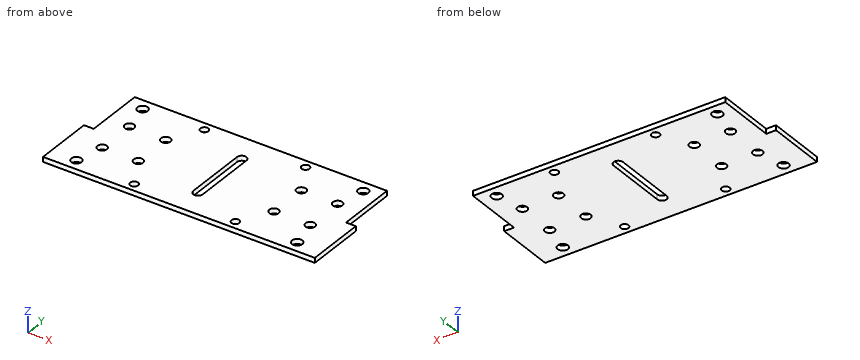
```python
from build123d import *

# Parameters (mm, degrees)
SKETCH1_W           = 160
SKETCH1_H           = 75
BOSS_EXTRUDE1_DEPTH = 3.1
SKETCH2_W           = 6.2
SKETCH2_H           = 37.5
BOSS_EXTRUDE2_DEPTH = 3.1
SKETCH3_R           = 2.5
SKETCH3_R_2         = 3
SKETCH3_R_3         = 3.25
CUT_EXTRUDE1_DEPTH  = 4.1


with BuildPart() as part:
    # Sketch1 → Boss-Extrude1 (new body)
    with BuildSketch(Plane.XY):
        Rectangle(SKETCH1_W, SKETCH1_H)
    extrude(amount=BOSS_EXTRUDE1_DEPTH)

    # Sketch2 → Boss-Extrude2 (add, through all)
    with BuildSketch(Plane.XY.offset(3.1)):
        with Locations((83.1, -18.75)):
            Rectangle(SKETCH2_W, SKETCH2_H)
        with Locations((-83.1, -18.75)):
            Rectangle(SKETCH2_W, SKETCH2_H)
    extrude(amount=-BOSS_EXTRUDE2_DEPTH)

    # Sketch3 → Cut-Extrude1 (cut, through all)
    with BuildSketch(Plane.XY.offset(3.1)):
        with Locations((32.08959236, 32.08959236)):
            Circle(SKETCH3_R)
        with Locations((32.08959236, -32.08959236)):
            Circle(SKETCH3_R)
        with Locations((-32.08959236, -32.08959236)):
            Circle(SKETCH3_R)
        with Locations((-32.08959236, 32.08959236)):
            Circle(SKETCH3_R)
        with Locations((-66, 12.5)):
            Circle(SKETCH3_R_2)
        with Locations((-43, 12.5)):
            Circle(SKETCH3_R_2)
        with Locations((-43, -12.5)):
            Circle(SKETCH3_R_2)
        with Locations((-66, -12.5)):
            Circle(SKETCH3_R_2)
        with Locations((43, 12.5)):
            Circle(SKETCH3_R_2)
        with Locations((66, 12.5)):
            Circle(SKETCH3_R_2)
        with Locations((66, -12.5)):
            Circle(SKETCH3_R_2)
        with Locations((43, -12.5)):
            Circle(SKETCH3_R_2)
        with Locations((-70, -30.258810311)):
            Circle(SKETCH3_R_3)
        with Locations((70, -30.258810311)):
            Circle(SKETCH3_R_3)
        with Locations((-70, 30.258810311)):
            Circle(SKETCH3_R_3)
        with Locations((70, 30.258810311)):
            Circle(SKETCH3_R_3)
        with BuildLine():
            Line((3, -20), (3, 20))
            ThreePointArc((3, 20), (0, 23), (-3, 20))
            Line((-3, 20), (-3, -20))
            ThreePointArc((-3, -20), (0, -23), (3, -20))
        make_face()
    extrude(amount=-CUT_EXTRUDE1_DEPTH, mode=Mode.SUBTRACT)


solid = part.part
```
The model under review builds one solid part; all positions refer to its coordinate system, in mm. Round coordinates to 2 decimals unless told otherwise and drop trailing zeros. Order: outer loops, then holes, each group sorted by start corner. A loop starts at its lowest first (then second) coordinate and runs counter-clockwise, first axis right, second up. Notation, with made-up numbers: M 36,-16 L 66,-16 A33 ccw 66,23 Z; hole C 26.5,30.5 d4. An arc over 180 degrees is marked long. Use a Markdown table: item, result.
1) Consider section C-C (z = 0.85). Give the number of separate pieces and of enclosed holes in the cut face, then the cut area to 3 significant figures.
Report:
| item | result |
|---|---|
| separate pieces | 1 |
| enclosed holes | 17 |
| area | 11,800 mm^2 |
2) Consider section B-B (x = 43). Write out the cut boundary in (y, z).
Report:
| item | result |
|---|---|
| outline | M -37.5,0 L -15.5,0 L -15.5,3.1 L -37.5,3.1 Z; M -9.5,0 L 9.5,0 L 9.5,3.1 L -9.5,3.1 Z; M 15.5,0 L 37.5,0 L 37.5,3.1 L 15.5,3.1 Z |
3) Consider section A-A (y = 12.5). Write out the cut boundary in (x, z), then the cut area to 3 significant figures.
Report:
| item | result |
|---|---|
| outline | M -80,0 L -69,0 L -69,3.1 L -80,3.1 Z; M -63,0 L -46,0 L -46,3.1 L -63,3.1 Z; M -40,0 L -3,0 L -3,3.1 L -40,3.1 Z; M 3,0 L 40,0 L 40,3.1 L 3,3.1 Z; M 46,0 L 63,0 L 63,3.1 L 46,3.1 Z; M 69,0 L 80,0 L 80,3.1 L 69,3.1 Z |
| area | 403 mm^2 |
4) Wall thickness on line 1 along Y through (x, z) = (-66, 1.2); line 2 along X through (y, z) = (-1, 1.65); line 3 along X through (y, z) = (17, 1.5): over which ranges is each line inside the solid? List them lowest first. Write a range as [from, to].
Report:
| item | result |
|---|---|
| line 1 | [-37.5, -15.5], [-9.5, 9.5], [15.5, 37.5] |
| line 2 | [-86.2, -3], [3, 86.2] |
| line 3 | [-80, -3], [3, 80] |
5) Insertion check: pin 1 (1 mm diameter, centred on y = 16.5, z = 1.5, fed in from +X). The pin has a flat end and moves straight along its axis. Give the tip position at first contact, or say it passes through.
Report:
| item | result |
|---|---|
| pin 1 | x = 80 |
